```python
from build123d import *

# Parameters (mm, degrees)
SALIENTE_EXTRUIR1_DEPTH                             = 20
CBORE_FOR_M2_HEX_SOCKET_HEAD_CAP_SCREW1_D           = 2.4
CBORE_FOR_M2_HEX_SOCKET_HEAD_CAP_SCREW1_CBORE_D     = 4.4
CBORE_FOR_M2_HEX_SOCKET_HEAD_CAP_SCREW1_CBORE_DEPTH = 2.4


with BuildPart() as part:
    # Croquis1 → Saliente-Extruir1 (new body)
    with BuildSketch(Plane(origin=(0, 0, 0), x_dir=(1, 0, 0), z_dir=(0, 1, 0))):
        Polygon((6.5, -10), (7.5, -10), (7.5, 10), (-7.5, 10), (-7.5, -10), (-6.5, -10), (-6.5, 9), (6.5, 9), align=None)
    extrude(amount=SALIENTE_EXTRUIR1_DEPTH)

    # CBORE for M2 Hex Socket Head Cap Screw1 (through all)
    with Locations(Plane.XY.offset(-9)):
        with Locations((0, 15)):
            CounterBoreHole(CBORE_FOR_M2_HEX_SOCKET_HEAD_CAP_SCREW1_D / 2, CBORE_FOR_M2_HEX_SOCKET_HEAD_CAP_SCREW1_CBORE_D / 2, CBORE_FOR_M2_HEX_SOCKET_HEAD_CAP_SCREW1_CBORE_DEPTH)


solid = part.part
```
Geometry: final body of the model. Coordinates: model frame, mm. A direction names the side the tool comes from. Coordinates: 2 decimals unless noted, no trailing zeros. Write each loop counter-clockwise with the first axis right and the second up, starting at its lowest first coordinate (ties: lowest second). Pieces come first, ordered by that corner, then holes. Notation, with made-up numbers: M 63.25,40.25 L 83.25,40.25 A15 ccw 83.25,62.25 Z; hole C 71,7.25 d6. An arc over 180 degrees is marked long. Use CSV: the item, a comma, the result in double quotes. Start each with the question number.
1. Cut plane A-A on y = 15. Return the cut outline in (x, z).
2. Cut plane C-C on x = 0. Return the cut outline in (y, z), plus the area to 3 significant figures.
3. Ray query, probe 1 along X at (y, z) = (6.5, 5); probe 2 along Y at (x, z) = (0, -9.7); probe 3 along Z at (x, y) = (1.5, 12.25). Return the intervals inside material, ascending.
4. Reachability of faces 4 (the face through (0, 10, -9)), 5 (the face through (-7.5, 10, 0)) from +Z, -Z, +X, -X, +Y, -Y: full face, straight path, thin tool, end or side. Return the list, or none.
5. Mould query, pull axis X, two halves, no side actions, for faces 1 (the face through (7.5, 10, 0)), 2 (the face through (-2.198, 15.097, -9.493)), 3 (the face through (0, 10, -10)). Classes: pulls with the +X half, pulls with the -X half, needs draft (parallel to the pull), parting line crosses it, or undercut.
6. Cut plane D-D on y = 18.75. Return the cut outline in (x, z).
7. First-contact query: P1, Ø5, axis at x = -2.5, y = 3.5, coming from the +Z side. Flat tip, straight axial feed; report the tip coordinate or a pass-through.
8. Cut plane B-B on z = -4.25. Return the cut outline in (x, y).
Entries:
1,outline,"M -7.5,-10 L -2.2,-10 L -2.2,-9 L -6.5,-9 L -6.5,10 L -7.5,10 Z; M 2.2,-10 L 7.5,-10 L 7.5,10 L 6.5,10 L 6.5,-9 L 2.2,-9 Z"
2,outline,"M 0,-10 L 12.8,-10 L 12.8,-9 L 0,-9 Z; M 17.2,-10 L 20,-10 L 20,-9 L 17.2,-9 Z"
2,area,"15.6 mm²"
3,probe 1,"-7.5 to -6.5, 6.5 to 7.5"
3,probe 2,"0 to 12.8, 17.2 to 20"
3,probe 3,"-10 to -9"
4,face 4,"+Z, +Y, -Y"
4,face 5,"+Z, -Z, -X, +Y, -Y"
5,face 1,"pulls with the +X half"
5,face 2,"undercut"
5,face 3,"needs draft"
6,outline,"M -7.5,-10 L 7.5,-10 L 7.5,10 L 6.5,10 L 6.5,-9 L -6.5,-9 L -6.5,10 L -7.5,10 Z"
7,P1,"z = -9"
8,outline,"M -7.5,0 L -6.5,0 L -6.5,20 L -7.5,20 Z; M 6.5,0 L 7.5,0 L 7.5,20 L 6.5,20 Z"
